Check sheet for the drawn part. Datum: minimum x, y, z corner. Units: mm. A direction names the side the tool comes from. Coordinates: 2 decimals unless noted, no trailing zeros. Write each loop counter-clockwise with the first axis right and the second up, starting at its lowest first coordinate (ties: lowest second). Pieces come first, ordered by that corner, then holes. Notation, with made-up numbers: (7.5, 64.25) -> (12.5, 64.25) arc R27 cw to (12.5, 102.25) -> close; hole circle Ø1 at (-8.75, -1.5). An arc over 180 degrees is marked (long way). Write each question's results on one line, items separated by ' | '. Start each with the question number.
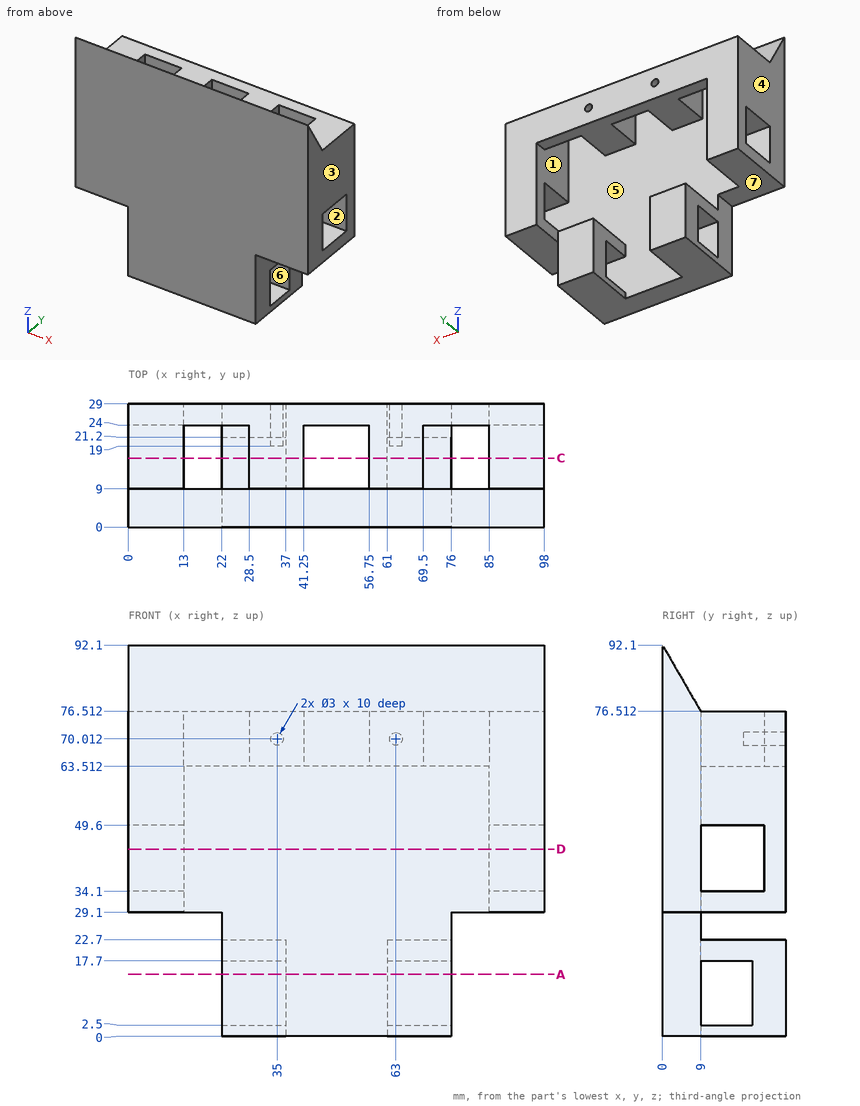
1. Sectioned sample at C-C on y = 16.25. State how many separate pieces and enclosed holes the cut face has, plus the area to 3 significant figures.
2. Material ranges on probe 1 along Z at (x, y) = (65, 10.5); probe 2 along X at (y, z) = (23.25, 18); probe 3 along Y at (x, z) = (18.5, 71), recorded low to high. Write a range as from..to.
3. Depth check by flat-ended pin: pin 1 Ø7.5 at (x, y) = (27.5, 17.5) entering from +Z; pin 2 Ø16 at (x, y) = (46.5, 19) entering from -Z; pin 3 Ø8.5 at (y, z) = (9.5, 20.5) entering from +X; pin 4 Ø6 at (y, z) = (14.5, 9) entering from +X. Enter the tip coordinate at first touch or a pass-through.
4. Sectioned sample at D-D on z = 44. Record the cut outline in (x, y).
5. Sectioned sample at A-A on z = 14.5. Record the cut outline in (x, y).
6. Tool access check on the marked faces 5, 6 and 7. Record the directions out of +Z, -Z, +X, -X, +Y, -Y that give a thin tool (end or side, any length) a straight path to the whole face; none if there is none.
7. Mould release check, pull along X, two halves, no side actions. Record for the marked faces 1, 2, 3 and 4: +X half, -X half, draft (parallel to the pull), parting line (faces both ways), or undercut.
Computed values:
1) separate pieces: 10 | enclosed holes: 0 | area: 1,390 mm^2
2) probe 1: z = 0..2.5, 17.7..22.7, 63.51..76.51 | probe 2: x = 22..37, 61..76 | probe 3: y = 0..9, 24..29
3) pin 1: stops at z = 76.51 | pin 2: stops at z = 63.51 | pin 3: stops at x = 76 | pin 4: passes through
4) outline: (0, 0) -> (98, 0) -> (98, 9) -> (0, 9) -> close; (0, 24) -> (13, 24) -> (13, 29) -> (0, 29) -> close; (85, 24) -> (98, 24) -> (98, 29) -> (85, 29) -> close
5) outline: (22, 0) -> (76, 0) -> (76, 9) -> (22, 9) -> close; (22, 21.2) -> (37, 21.2) -> (37, 29) -> (22, 29) -> close; (61, 21.2) -> (76, 21.2) -> (76, 29) -> (61, 29) -> close
6) face 5: none | face 6: +X, -X | face 7: -Z, -X, +Y, -Y
7) face 1: undercut | face 2: draft | face 3: +X half | face 4: -X half
